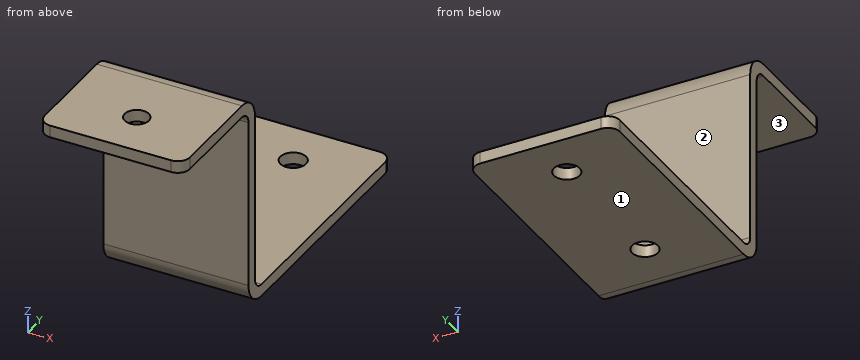
from build123d import *

# Parameters (mm, degrees)
SKETCH1_W                    = 38.1
SKETCH1_H                    = 57.15
BASE_FLANGE1_DEPTH           = 3.175
EDGE_FLANGE1_STRIP_W         = 19.05
EDGE_FLANGE1_STRIP_H         = 3.175
EDGE_FLANGE1_STRIP_CUT_DEPTH = 38.1
EDGE_FLANGE1_DEPTH           = 38.1
EDGE_FLANGE2_STRIP_W         = 19.05
EDGE_FLANGE2_STRIP_H         = 3.175
EDGE_FLANGE2_STRIP_CUT_DEPTH = 38.1
EDGE_FLANGE2_DEPTH           = 38.1
F_1_4_CLEARANCE_HOLE1_D      = 6.7564
F_1_4_20_TAPPED_HOLE1_D      = 6.35
BREAK_CORNER1_START          = -57.15
BREAK_CORNER1_DEPTH          = 57.15


# Read off the part's stored shape, not the designer's step: Break-Corner1
# Sheet-metal steps are written as plain solids
with BuildPart() as part:
    # Sketch1 → Base-Flange1 (new body)
    with BuildSketch(Plane(origin=(0, 0, 0), x_dir=(1, 0, 0), z_dir=(0, 1, 0))):
        with Locations((19.05, 28.575)):
            Rectangle(SKETCH1_W, SKETCH1_H)
    extrude(amount=-BASE_FLANGE1_DEPTH)

    # Edge-Flange1 strip (across the edge) → Edge-Flange1 strip cut (cut)
    with BuildSketch(Plane(origin=(38.1, 0, -57.15), x_dir=(0, 0, 1), z_dir=(-1, 0, 0))):
        with Locations((-3.175, -1.5875)):
            Rectangle(EDGE_FLANGE1_STRIP_W, EDGE_FLANGE1_STRIP_H)
    extrude(amount=EDGE_FLANGE1_STRIP_CUT_DEPTH, mode=Mode.SUBTRACT)

    # Edge-Flange1 section (across the edge) → Edge-Flange1 (add)
    with BuildSketch(Plane(origin=(38.1, 0, -57.15), x_dir=(0, 0, 1), z_dir=(-1, 0, 0))):
        with BuildLine():
            Line((0, 3.175), (0, 66.675))
            Line((0, 66.675), (3.175, 66.675))
            Line((3.175, 66.675), (3.175, 3.175))
            ThreePointArc((3.175, 3.175), (4.10493597, 0.92993597), (6.35, 0))
            Line((6.35, 0), (6.35, -3.175))
            ThreePointArc((6.35, -3.175), (1.859871939, -1.315128061), (0, 3.175))
        make_face()
    extrude(amount=EDGE_FLANGE1_DEPTH)

    # Edge-Flange2 strip (across the edge) → Edge-Flange2 strip cut (cut)
    with BuildSketch(Plane(origin=(38.1, -3.175, 0), x_dir=(0, 0, -1), z_dir=(-1, 0, 0))):
        with Locations((-3.175, -1.5875)):
            Rectangle(EDGE_FLANGE2_STRIP_W, EDGE_FLANGE2_STRIP_H)
    extrude(amount=EDGE_FLANGE2_STRIP_CUT_DEPTH, mode=Mode.SUBTRACT)

    # Edge-Flange2 section (across the edge) → Edge-Flange2 (add)
    with BuildSketch(Plane(origin=(38.1, -3.175, 0), x_dir=(0, 0, -1), z_dir=(-1, 0, 0))):
        with BuildLine():
            Line((0, 3.175), (0, 31.75))
            Line((0, 31.75), (3.175, 31.75))
            Line((3.175, 31.75), (3.175, 3.175))
            ThreePointArc((3.175, 3.175), (4.10493597, 0.92993597), (6.35, 0))
            Line((6.35, 0), (6.35, -3.175))
            ThreePointArc((6.35, -3.175), (1.859871939, -1.315128061), (0, 3.175))
        make_face()
    extrude(amount=EDGE_FLANGE2_DEPTH)

    # 1/4 Clearance Hole1 (through all)
    with Locations(Plane.XY.offset(-53.975)):
        with Locations((19.05, 53.975), (19.05, 15.875)):
            Hole(F_1_4_CLEARANCE_HOLE1_D / 2)

    # 1/4-20 Tapped Hole1 (through all)
    with Locations(Plane.XY):
        with Locations((19.05, -22.225)):
            Hole(F_1_4_20_TAPPED_HOLE1_D / 2)

    # Break-Corner1 outline → Break-Corner1 (cut)
    with BuildSketch(Plane.XY.offset(BREAK_CORNER1_START)):
        with BuildLine():
            Line((38.1, -34.925), (38.1, -31.75))
            ThreePointArc((38.1, -31.75), (37.17006403, -33.99506403), (34.925, -34.925))
            Line((34.925, -34.925), (38.1, -34.925))
        make_face()
        with BuildLine():
            Line((0, -34.925), (3.175, -34.925))
            ThreePointArc((3.175, -34.925), (0.92993597, -33.99506403), (0, -31.75))
            Line((0, -31.75), (0, -34.925))
        make_face()
        with BuildLine():
            ThreePointArc((0, 63.5), (0.92993597, 65.74506403), (3.175, 66.675))
            Line((3.175, 66.675), (0, 66.675))
            Line((0, 66.675), (0, 63.5))
        make_face()
        with BuildLine():
            ThreePointArc((34.925, 66.675), (37.17006403, 65.74506403), (38.1, 63.5))
            Line((38.1, 63.5), (38.1, 66.675))
            Line((38.1, 66.675), (34.925, 66.675))
        make_face()
    extrude(amount=BREAK_CORNER1_DEPTH, mode=Mode.SUBTRACT)


solid = part.part
For this review, take the finished solid that the model builds, in its own axes (mm). Face numbers are marked on the shaded views. A direction names the side the tool comes from. Round coordinates to 2 decimals unless told otherwise and drop trailing zeros. Order: outer loops, then holes, each group sorted by start corner. A loop starts at its lowest first (then second) coordinate and runs counter-clockwise, first axis right, second up. Notation, with made-up numbers: (64, -26) -> (72, -26) arc R27 ccw to (72, 11) -> close; hole circle Ø7 at (70.5, 7.25). An arc over 180 degrees is marked (long way). Put each result on its own line as item: value.
Q1. Insertion check: pin 1 Ø1 at (x, z) = (22, -27) entering from -Y (3 decimals); pin 2 Ø5.5 at (x, y) = (19.05, 53.975) entering from -Z; pin 3 Ø14.5 at (x, y) = (28, -20.5) entering from -Z (3 decimals); pin 4 Ø1 at (x, y) = (16.5, 37) entering from +Z (3 decimals). Each pin has a flat end and moves straight along its axis. Give the tip position at first contact, or say it passes through.
Check result:
pin 1: y = -3.175
pin 2: through
pin 3: z = -3.175
pin 4: z = -53.975
Q2. Add section A-A on x = 19.05. Write out the cut boundary in (y, z) (3 decimals), plus the area to 3 significant figures.
Check result:
outline: (-34.925, -3.175) -> (-25.4, -3.175) -> (-25.4, 0) -> (-34.925, 0) -> close; (-19.05, -3.175) -> (-6.35, -3.175) arc R3.175 cw to (-3.175, -6.35) -> (-3.175, -50.8) arc R6.35 ccw to (3.175, -57.15) -> (12.497, -57.15) -> (12.497, -53.975) -> (3.175, -53.975) arc R3.175 cw to (0, -50.8) -> (0, -6.35) arc R6.35 ccw to (-6.35, 0) -> (-19.05, 0) -> close; (19.253, -57.15) -> (50.597, -57.15) -> (50.597, -53.975) -> (19.253, -53.975) -> close; (57.353, -57.15) -> (66.675, -57.15) -> (66.675, -53.975) -> (57.353, -53.975) -> close
area: 418 mm2
Q3. Machinability: for the marked faces 1, 2 and 3, which of the approach directions +Z, -Z, +X, -X, +Y, -Y give a long, thin tool a straight path to every point of the face, cutting with its end or side? Answer none if there is none.
Check result:
face 1: -Z, +X, -X, +Y, -Y
face 2: +Z, +X, -X, +Y
face 3: -Z, +X, -X, -Y
Q4. Add section C-C on x = 11.5. Write out the cut boundary in (y, z) (3 decimals).
Check result:
outline: (-34.925, -3.175) -> (-6.35, -3.175) arc R3.175 cw to (-3.175, -6.35) -> (-3.175, -50.8) arc R6.35 ccw to (3.175, -57.15) -> (66.675, -57.15) -> (66.675, -53.975) -> (3.175, -53.975) arc R3.175 cw to (0, -50.8) -> (0, -6.35) arc R6.35 ccw to (-6.35, 0) -> (-34.925, 0) -> close
Q5. Add section B-B on y = 55. Write out the cut boundary in (x, z) (3 decimals), plus the area to 3 significant figures.
Check result:
outline: (0, -57.15) -> (15.831, -57.15) -> (15.831, -53.975) -> (0, -53.975) -> close; (22.269, -57.15) -> (38.1, -57.15) -> (38.1, -53.975) -> (22.269, -53.975) -> close
area: 101 mm2
Q6. For probe 1 along Y at (x, z) = (19, -56) (3 decimals); probe 2 along Z at (x, y) = (5.5, 40) (3 decimals); probe 3 along Y at (x, z) = (5.5, -41) (3 decimals), list the stretches that pass through material, from the lowest coordinate up. Write a range as [from, to].
Check result:
probe 1: [-0.47, 12.497], [19.253, 50.597], [57.353, 66.675]
probe 2: [-57.15, -53.975]
probe 3: [-3.175, 0]
Q7. Add section D-D on y = -28. Write out the cut boundary in (x, z) (3 decimals), plus the area to 3 significant figures.
Check result:
outline: (0, -3.175) -> (38.1, -3.175) -> (38.1, 0) -> (0, 0) -> close
area: 121 mm2
